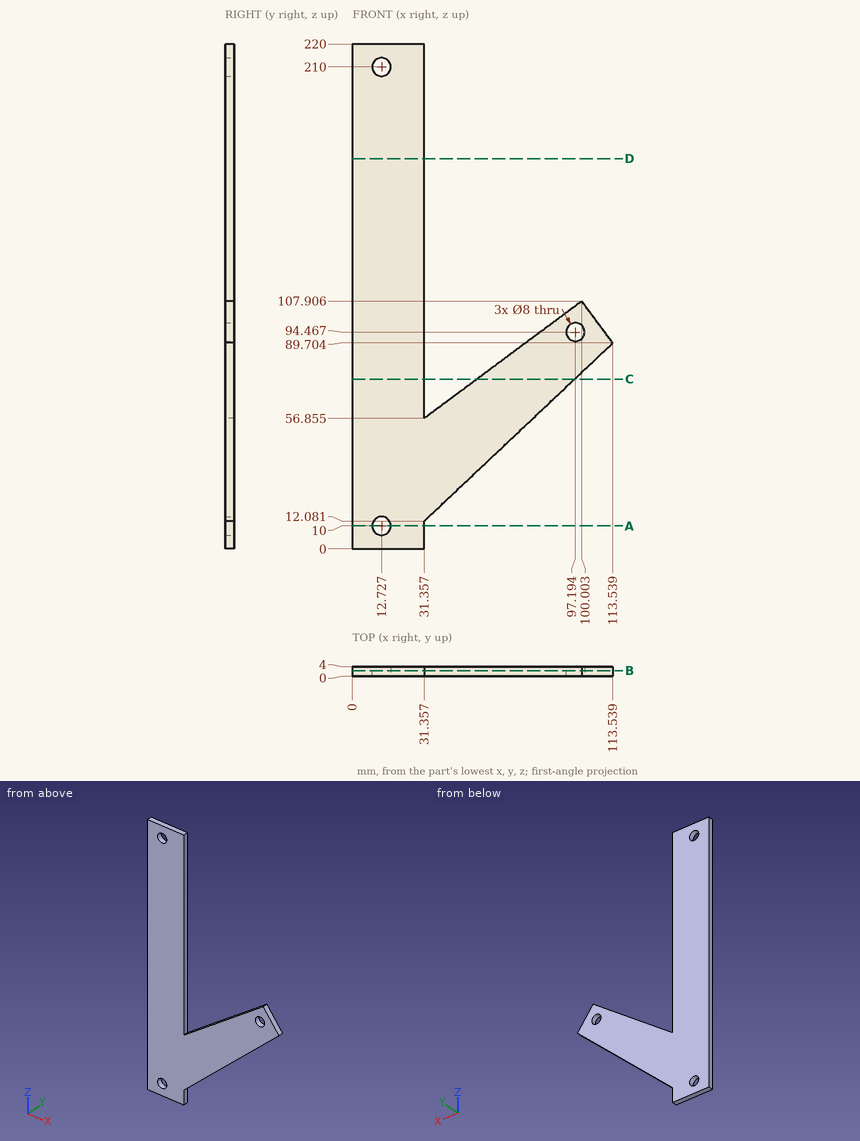
Input: dimensioned drawing with shaded views. Units: mm. Origin: part minimum x, y, z. Round coordinates to 2 decimals unless told otherwise and drop trailing zeros. Loops run counter-clockwise (first coordinate to the right, second up) from the corner with the lowest first, then second, coordinate; pieces in that order, holes last. Notation, with made-up numbers: M 37,29.5 L 66,29.5 A33 cw 66,62.5 Z; hole C 61,23.5 d11. An arc over 180 degrees is marked long. One line per question, with ' | ' between items.
(1) Cut plane D-D on z = 170. Return the cut outline in (x, y), plus the area to 3 significant figures.
Check result:
outline: M 0,0 L 31.36,0 L 31.36,4 L 0,4 Z | area: 125 mm2
(2) Cut plane C-C on z = 74. Return the cut outline in (x, y).
Check result:
outline: M 0,0 L 31.36,0 L 31.36,4 L 0,4 Z; M 54.41,0 L 96.91,0 L 96.91,4 L 54.41,4 Z
(3) Cut plane A-A on z = 10. Return the cut outline in (x, y).
Check result:
outline: M 0,0 L 8.73,0 L 8.73,4 L 0,4 Z; M 16.73,0 L 31.36,0 L 31.36,4 L 16.73,4 Z
(4) Material intervals for line 1 along X through (y, z) = (2.2, 97.5) (1 decimal); line 2 along X through (y, z) = (2.75, 73) (1 decimal); line 3 along X through (y, z) = (0.25, 100.5) (1 decimal), sorted ascending. Write a range as from..to.
Check result:
line 1: x = 0..31.4, 86..94.6, 99.8..107.7 | line 2: x = 0..31.4, 53.1..95.9 | line 3: x = 0..31.4, 90..105.5
(5) Contact query for flat-ended pins moving along their axis: P1, Ø2, axis at y = 2, z = 147, coming from the +X side; P2, Ø5, axis at x = 12.73, z = 210, coming from the -Y side. Output: stop coordinate, or through.
Check result:
P1: stops at x = 31.36 | P2: passes through
(6) Cut plane B-B on y = 2.35. Return the cut outline in (x, z) (1 decimal).
Check result:
outline: M 0,0 L 31.4,0 L 31.4,12.1 L 113.5,89.7 L 100,107.9 L 31.4,56.9 L 31.4,220 L 0,220 Z; hole C 12.7,10 d8; hole C 12.7,210 d8; hole C 97.2,94.5 d8
